Source: CAD feature listing. Evaluate the final solid. Frame: model axes, mm. Coordinates: 2 decimals unless noted, no trailing zeros. Order: outer loops, then holes, each group sorted by start corner. A loop starts at its lowest first (then second) coordinate and runs counter-clockwise, first axis right, second up.
```python
from build123d import *

# Parameters (mm, degrees)
SKETCH1_R           = 2.05
SKETCH1_R_2         = 7
BOSS_EXTRUDE1_DEPTH = 3.175


with BuildPart() as part:
    # Sketch1 → Boss-Extrude1 (new body)
    with BuildSketch(Plane(origin=(0, 0, 0), x_dir=(1, 0, 0), z_dir=(0, 1, 0))):
        with BuildLine():
            Line((-16, 122.55), (-16, 112.55))
            ThreePointArc((-16, 112.55), (25.275, 71.275), (-16, 30))
            Line((-16, 30), (-16, 0))
            ThreePointArc((-16, 0), (0, -16), (16, 0))
            ThreePointArc((16, 0), (8.94427191, 13.266499161), (-6, 14.832396974))
            Line((-6, 14.832396974), (-6, 20))
            ThreePointArc((-6, 20), (35.518206733, 75.811148877), (-16, 122.55))
        make_face()
        with Locations(Location((-8, 8, 0), (0, 0, 270))):
            Circle(SKETCH1_R, mode=Mode.SUBTRACT)
        with Locations(Location((8, 8, 0), (0, 0, 270))):
            Circle(SKETCH1_R, mode=Mode.SUBTRACT)
        with Locations(Location((8, -8, 0), (0, 0, 270))):
            Circle(SKETCH1_R, mode=Mode.SUBTRACT)
        with Locations(Location((-8, -8, 0), (0, 0, 270))):
            Circle(SKETCH1_R, mode=Mode.SUBTRACT)
        with Locations(Location((-11, 25, 0), (0, 0, 270))):
            Circle(SKETCH1_R, mode=Mode.SUBTRACT)
        with Locations(Location((-11, 117.55, 0), (0, 0, 90))):
            Circle(SKETCH1_R, mode=Mode.SUBTRACT)
        with Locations(Location((0, 0, 0), (0, 0, 270))):
            Circle(SKETCH1_R_2, mode=Mode.SUBTRACT)
    extrude(amount=BOSS_EXTRUDE1_DEPTH)


solid = part.part
```
1. Section query A-A, the plane y = 0.85. Output: boundary loops of the cut face in (x, z) (3 decimals), plus the area to 3 significant figures.
2. Section query B-B, the plane z = -117.55. Output: boundary loops of the cut face in (x, y) (3 decimals), plus the area to 3 significant figures.
3. Contact query for a flat-ended pin moving along its axis: P1, Ø1.6, axis at y = 2, z = -17.5, coming from the +X side. Output: stop coordinate, or through.
4. Material intervals for line 1 along Z through (x, y) = (4.5, 1.05); line 2 along X through (y, z) = (2.7, -8); line 3 along Z through (x, y) = (-3.5, 0.5), sorted ascending.
5. Section query D-D, the plane z = -64.5. Output: boundary loops of the cut face in (x, y) (3 decimals), plus the area to 3 significant figures.
6. Section query C-C, the plane x = 23. Output: boundary loops of the cut face in (y, z) (3 decimals).
7. Draft query along Z for faces 1 (the cylindrical face through (-7.91, 1.57, -10.05)), 2 (the flat face through (16, 3.175, -43)). Return one class per face: +Z half, -Z half, draft (parallel to the pull), parting line (faces both ways), or undercut.
Answer key:
1. outline: (-16, -122.55) arc R51.763 ccw to (-6, -20) - (-6, -14.832) arc R16 ccw (long way) to (-16, 0) - (-16, -30) arc R41.275 cw to (-16, -112.55) - close; hole circle Ø4.1 at (-11, -117.55); hole circle Ø4.1 at (-11, -25); hole circle Ø4.1 at (-8, -8); hole circle Ø4.1 at (-8, 8); hole circle Ø14 at (0, 0); hole circle Ø4.1 at (8, -8); hole circle Ø4.1 at (8, 8)
1. area: 2,190 mm2
2. outline: (-16, 0) - (-13.05, 0) - (-13.05, 3.175) - (-16, 3.175) - close; (-8.95, 0) - (6.195, 0) - (6.195, 3.175) - (-8.95, 3.175) - close
2. area: 57.5 mm2
3. P1: stops at x = -6
4. line 1: z = -118.32 to -107.1, -35.45 to -23.26, -15.35 to -5.36, 5.36 to 15.35
4. line 2: x = -16 to -10.05, -5.95 to 5.95, 10.05 to 13.86
4. line 3: z = -121.02 to -110.61, -31.94 to -20.56, -15.61 to -6.06, 6.06 to 15.61
5. outline: (24.715, 0) - (35.379, 0) - (35.379, 3.175) - (24.715, 3.175) - close
5. area: 33.9 mm2
6. outline: (0, -104.822) - (3.175, -104.822) - (3.175, -84.789) - (0, -84.789) - close; (0, -57.761) - (3.175, -57.761) - (3.175, -36.753) - (0, -36.753) - close
7. face 1: undercut
7. face 2: draft
